Can you work these out from the model? Positions are in its coordinate system, mm. A direction names the side the tool comes from. Round coordinates to 2 decimals unless told otherwise and drop trailing zeros. Loops run counter-clockwise (first coordinate to the right, second up) from the corner with the lowest first, then second, coordinate; pieces in that order, holes last.
from build123d import *

# Parameters (mm, degrees)
F0_W     = 26.747306
F0_H     = 25
F1_DEPTH = 35
F2_W     = 4.5
F2_H     = 20
F3_DEPTH = 20
F4_W     = 19.263828
F4_H     = 4
F5_DEPTH = 20
F6_W     = 23
F6_H     = 4.5
F7_DEPTH = 20


with BuildPart() as f1:
    # F0 (on Top) → F1 (new body)
    with BuildSketch(Plane.XY):
        Rectangle(F0_W, F0_H)
    extrude(amount=F1_DEPTH)

    # F2 (on face) → F3 (cut)
    with BuildSketch(Plane.XY.offset(35)):
        with Locations((-7.640175, -2.5)):
            Rectangle(F2_W, F2_H)
    extrude(amount=-F3_DEPTH, mode=Mode.SUBTRACT)

    # F4 (on face) → F5 (cut)
    with BuildSketch(Plane.XY.offset(35)):
        with Locations((3.741739, 5.5)):
            Rectangle(F4_W, F4_H)
    extrude(amount=-F5_DEPTH, mode=Mode.SUBTRACT)

    # F6 (on face) → F7 (cut)
    with BuildSketch(Plane.XZ.offset(12.5)):
        with Locations((1.873653, 6.339478)):
            Rectangle(F6_W, F6_H)
    extrude(amount=-F7_DEPTH, mode=Mode.SUBTRACT)


solid = f1.part
(1) If I drill on line 1 (Y direction, x = 1, z = 29.5); line 2 (Z direction, x = 0.25, y = -6.5); line 3 (X direction, y = -6.75, z = 15.5), over which ranges is the centre line in solid material (lowest first)?
Worked answers:
line 1: y = -12.5 to 3.5, 7.5 to 12.5
line 2: z = 0 to 4.09, 8.59 to 35
line 3: x = -13.37 to -9.89, -5.39 to 13.37
(2) If we section it at A-A, the plane z = 16: List the corners of the cut face in (x, y) for me, then the cut area to 3 significant figures.
Worked answers:
outline: (-13.37, -12.5) - (-9.89, -12.5) - (-9.89, 7.5) - (13.37, 7.5) - (13.37, 12.5) - (-13.37, 12.5) - close; (-5.39, -12.5) - (13.37, -12.5) - (13.37, 3.5) - (-5.39, 3.5) - close
area: 504 mm2
(3) If we mould it in two halves opening along Z, with no side actions, what happens to faces 1 (the flat face through (2, -3, 4.089)), 2 (the flat face through (2, 7.5, 25)), 3 (the flat face through (-5, 9, 35)), 4 (the flat face through (0, 0, 0))? For each: released by +Z, released by -Z, zero draft, split by the parting line, or undercut.
Worked answers:
face 1: undercut
face 2: zero draft
face 3: released by +Z
face 4: released by -Z
(4) If we section it at B-B, the plane y = -3: List the corners of the cut face in (x, z) for me, then the cut area to 3 significant figures.
Worked answers:
outline: (-13.37, 0) - (13.37, 0) - (13.37, 4.09) - (-9.63, 4.09) - (-9.63, 8.59) - (13.37, 8.59) - (13.37, 35) - (-5.39, 35) - (-5.39, 15) - (-9.89, 15) - (-9.89, 35) - (-13.37, 35) - close
area: 743 mm2
(5) For faces 5 (the flat face through (2, -3, 8.589)), 6 (the flat face through (4, 3.5, 25)), 7 (the flat face through (0, 12.5, 17)), 8 (the flat face through (-5.39, -5, 25)), which set-ups out of +Z, -Z, +X, -X, +Y, -Y let a thin tool reach every point of the face, with its end or its side?
Worked answers:
face 5: +X, -Y
face 6: +Z, +X
face 7: +Z, -Z, +X, -X, +Y
face 8: +Z, -Y
(6) If we section it at C-C, the plane x = -4.25: List the corners of the cut face in (y, z) for me, then the cut area to 3 significant figures.
Worked answers:
outline: (-12.5, 0) - (12.5, 0) - (12.5, 35) - (7.5, 35) - (7.5, 15) - (3.5, 15) - (3.5, 35) - (-12.5, 35) - (-12.5, 8.59) - (7.5, 8.59) - (7.5, 4.09) - (-12.5, 4.09) - close
area: 705 mm2
(7) If we section it at D-D, the plane z = 5.5: List the corners of the cut face in (x, y) for me.
Worked answers:
outline: (-13.37, -12.5) - (-9.63, -12.5) - (-9.63, 7.5) - (13.37, 7.5) - (13.37, 12.5) - (-13.37, 12.5) - close
(8) Will this pin go through, and if not, where does the flat tip stop? P1, Ø1.3, axis at x = -2, z = 6, coming from the -Y side.
Worked answers:
P1: stops at y = 7.5
